```python
from build123d import *

# Parameters (mm, degrees)
EXTRUDE_THIN1_DEPTH = 4
SKETCH2_R           = 1.5
BOSS_EXTRUDE1_DEPTH = 4
FILLET1_DEPTH       = 4
FILLET1_2_DEPTH     = 4
SKETCH3_W           = 3.133113898
SKETCH3_H           = 7.459824135
CUT_EXTRUDE1_DEPTH  = 95.769370322


with BuildPart() as part:
    # Sketch1 → Extrude-Thin1 (new body)
    with BuildSketch(Plane.XY):
        Polygon((-70, -25.358547654), (30, 11.038475773), (-60, 63), (-70, 63), (-70, 61), (-60.535898385, 61), (25.285605056, 11.450931886), (-70.684040287, -23.479162412), align=None)
    extrude(amount=EXTRUDE_THIN1_DEPTH)

    # Sketch2 → Boss-Extrude1 (add)
    # profile 1 of 17: a face of its own
    with BuildSketch(Plane(origin=(0, 0, 0), x_dir=(-1, 0, 0), z_dir=(0, 0, -1))):
        with BuildLine():
            ThreePointArc((69.699771159, -19.718666382), (66.807539781, -16.271839247), (62.910846986, -18.521595881))
            ThreePointArc((62.910846986, -18.521595881), (62.703305352, -19.561418618), (62.816669308, -20.615673554))
            Line((62.816669308, -20.615673554), (68.214792437, -22.580429694))
            ThreePointArc((68.214792437, -22.580429694), (68.979296275, -21.845692505), (69.488695332, -20.915736884))
            ThreePointArc((69.488695332, -20.915736884), (69.646598295, -20.326435004), (69.699771159, -19.718666382))
        make_face()
        with Locations((66.199771159, -19.718666382)):
            Circle(SKETCH2_R, mode=Mode.SUBTRACT)
    # profile 2 of 17: a face of its own
    with BuildSketch(Plane(origin=(0, 0, 0), x_dir=(-1, 0, 0), z_dir=(0, 0, -1))):
        with BuildLine():
            ThreePointArc((69.488695332, -20.915736884), (68.979296275, -21.845692505), (68.214792437, -22.580429694))
            Line((68.214792437, -22.580429694), (68.804655045, -22.795122125))
            Line((68.804655045, -22.795122125), (69.488695332, -20.915736884))
        make_face()
    # profile 3 of 17: a face of its own
    with BuildSketch(Plane(origin=(0, 0, 0), x_dir=(-1, 0, 0), z_dir=(0, 0, -1))):
        with BuildLine():
            Line((62.910846986, -18.521595881), (62.2268067, -20.400981122))
            Line((62.2268067, -20.400981122), (62.816669308, -20.615673554))
            ThreePointArc((62.816669308, -20.615673554), (62.703305352, -19.561418618), (62.910846986, -18.521595881))
        make_face()
    # profile 4 of 17: a face of its own
    with BuildSketch(Plane(origin=(0, 0, 0), x_dir=(-1, 0, 0), z_dir=(0, 0, -1))):
        with BuildLine():
            ThreePointArc((22.71514012, -2.617659216), (19.822908742, 0.82916792), (15.926215947, -1.420588714))
            ThreePointArc((15.926215947, -1.420588714), (15.718674313, -2.460411452), (15.832038269, -3.514666388))
            Line((15.832038269, -3.514666388), (21.230161397, -5.479422527))
            ThreePointArc((21.230161397, -5.479422527), (21.994665236, -4.744685339), (22.504064292, -3.814729718))
            ThreePointArc((22.504064292, -3.814729718), (22.661967255, -3.225427838), (22.71514012, -2.617659216))
        make_face()
        with Locations((19.21514012, -2.617659216)):
            Circle(SKETCH2_R, mode=Mode.SUBTRACT)
    # profile 5 of 17: a face of its own
    with BuildSketch(Plane(origin=(0, 0, 0), x_dir=(-1, 0, 0), z_dir=(0, 0, -1))):
        with BuildLine():
            ThreePointArc((22.504064292, -3.814729718), (21.994665236, -4.744685339), (21.230161397, -5.479422527))
            Line((21.230161397, -5.479422527), (21.820024006, -5.694114959))
            Line((21.820024006, -5.694114959), (22.504064292, -3.814729718))
        make_face()
    # profile 6 of 17: a face of its own
    with BuildSketch(Plane(origin=(0, 0, 0), x_dir=(-1, 0, 0), z_dir=(0, 0, -1))):
        with BuildLine():
            Line((15.926215947, -1.420588714), (15.24217566, -3.299973956))
            Line((15.24217566, -3.299973956), (15.832038269, -3.514666388))
            ThreePointArc((15.832038269, -3.514666388), (15.718674313, -2.460411452), (15.926215947, -1.420588714))
        make_face()
    # profile 7 of 17: a face of its own
    with BuildSketch(Plane(origin=(0, 0, 0), x_dir=(-1, 0, 0), z_dir=(0, 0, -1))):
        with BuildLine():
            ThreePointArc((-18.249808849, 11.760273971), (-18.650603728, 13.386597315), (-19.761196061, 14.640450906))
            Line((-19.761196061, 14.640450906), (-22.499808851, 13.059312075))
            ThreePointArc((-22.499808851, 13.059312075), (-20.99980885, 13.059312077), (-20.249808849, 11.760273971))
            ThreePointArc((-20.249808849, 11.760273971), (-20.889444174, 10.531545919), (-22.262839017, 10.350735022))
            Line((-22.262839017, 10.350735022), (-19.291270082, 9.269172381))
            ThreePointArc((-19.291270082, 9.269172381), (-18.520653721, 10.410252801), (-18.249808849, 11.760273971))
        make_face()
    # profile 8 of 17: a face of its own
    with BuildSketch(Plane(origin=(0, 0, 0), x_dir=(-1, 0, 0), z_dir=(0, 0, -1))):
        with BuildLine():
            Line((-22.499808851, 13.059312075), (-25.238421636, 11.478173246))
            ThreePointArc((-25.238421636, 11.478173246), (-25.236490292, 11.455228871), (-25.234408046, 11.432297698))
            Line((-25.234408046, 11.432297698), (-22.262839017, 10.350735022))
            ThreePointArc((-22.262839017, 10.350735022), (-23.244100894, 11.62954033), (-22.499808851, 13.059312075))
        make_face()
    # profile 9 of 17: a face of its own
    with BuildSketch(Plane(origin=(0, 0, 0), x_dir=(-1, 0, 0), z_dir=(0, 0, -1))):
        with BuildLine():
            ThreePointArc((-18.249808849, 11.760273971), (-18.650603728, 13.386597315), (-19.761196061, 14.640450906))
            Line((-19.761196061, 14.640450906), (-22.499808851, 13.059312075))
            ThreePointArc((-22.499808851, 13.059312075), (-20.99980885, 13.059312077), (-20.249808849, 11.760273971))
            ThreePointArc((-20.249808849, 11.760273971), (-20.889444174, 10.531545919), (-22.262839017, 10.350735022))
            Line((-22.262839017, 10.350735022), (-19.291270082, 9.269172381))
            ThreePointArc((-19.291270082, 9.269172381), (-18.520653721, 10.410252801), (-18.249808849, 11.760273971))
        make_face()
    # profile 10 of 17: a face of its own
    with BuildSketch(Plane(origin=(0, 0, 0), x_dir=(-1, 0, 0), z_dir=(0, 0, -1))):
        with BuildLine():
            Line((-22.499808851, 13.059312075), (-25.238421636, 11.478173246))
            ThreePointArc((-25.238421636, 11.478173246), (-25.236490292, 11.455228871), (-25.234408046, 11.432297698))
            Line((-25.234408046, 11.432297698), (-22.262839017, 10.350735022))
            ThreePointArc((-22.262839017, 10.350735022), (-23.244100894, 11.62954033), (-22.499808851, 13.059312075))
        make_face()
    # profile 11 of 17: a face of its own
    with BuildSketch(Plane(origin=(0, 0, 0), x_dir=(-1, 0, 0), z_dir=(0, 0, -1))):
        with BuildLine():
            ThreePointArc((-25.234408046, 11.432297698), (-25.236490292, 11.455228871), (-25.238421636, 11.478173246))
            Line((-25.238421636, 11.478173246), (-25.285605056, 11.450931886))
            Line((-25.285605056, 11.450931886), (-25.234408046, 11.432297698))
        make_face()
    # profile 12 of 17: a face of its own
    with BuildSketch(Plane(origin=(0, 0, 0), x_dir=(-1, 0, 0), z_dir=(0, 0, -1))):
        with BuildLine():
            ThreePointArc((27.36379332, 37.517949192), (27.244533712, 38.42381585), (26.894882233, 39.267949192))
            ThreePointArc((26.894882233, 39.267949192), (26.231736995, 40.09532048), (25.351261913, 40.686140662))
            Line((25.351261913, 40.686140662), (20.376324727, 37.813859338))
            ThreePointArc((20.376324727, 37.813859338), (20.447752473, 36.75593546), (20.832704407, 35.767949192))
            ThreePointArc((20.832704407, 35.767949192), (24.769659978, 34.1372088), (27.36379332, 37.517949192))
        make_face()
        with Locations((23.86379332, 37.517949192)):
            Circle(SKETCH2_R, mode=Mode.SUBTRACT)
    # profile 13 of 17: a face of its own
    with BuildSketch(Plane(origin=(0, 0, 0), x_dir=(-1, 0, 0), z_dir=(0, 0, -1))):
        with BuildLine():
            Line((26.894882233, 39.267949192), (25.894882233, 41))
            Line((25.894882233, 41), (25.351261913, 40.686140662))
            ThreePointArc((25.351261913, 40.686140662), (26.231736995, 40.09532048), (26.894882233, 39.267949192))
        make_face()
    # profile 14 of 17: a face of its own
    with BuildSketch(Plane(origin=(0, 0, 0), x_dir=(-1, 0, 0), z_dir=(0, 0, -1))):
        with BuildLine():
            ThreePointArc((20.832704407, 35.767949192), (20.447752473, 36.75593546), (20.376324727, 37.813859338))
            Line((20.376324727, 37.813859338), (19.832704407, 37.5))
            Line((19.832704407, 37.5), (20.832704407, 35.767949192))
        make_face()
    # profile 15 of 17: a face of its own
    with BuildSketch(Plane(origin=(0, 0, 0), x_dir=(-1, 0, 0), z_dir=(0, 0, -1))):
        with BuildLine():
            ThreePointArc((61, 59), (64.5, 55.5), (68, 59))
            ThreePointArc((68, 59), (67.839385021, 60.048097173), (67.372281323, 61))
            Line((67.372281323, 61), (61.627718677, 61))
            ThreePointArc((61.627718677, 61), (61.160614979, 60.048097173), (61, 59))
        make_face()
        with Locations((64.5, 59)):
            Circle(SKETCH2_R, mode=Mode.SUBTRACT)
    # profile 16 of 17: a face of its own
    with BuildSketch(Plane(origin=(0, 0, 0), x_dir=(-1, 0, 0), z_dir=(0, 0, -1))):
        with BuildLine():
            Line((61, 61), (61, 59))
            ThreePointArc((61, 59), (61.160614979, 60.048097173), (61.627718677, 61))
            Line((61.627718677, 61), (61, 61))
        make_face()
    # profile 17 of 17: a face of its own
    with BuildSketch(Plane(origin=(0, 0, 0), x_dir=(-1, 0, 0), z_dir=(0, 0, -1))):
        with BuildLine():
            ThreePointArc((67.372281323, 61), (67.839385021, 60.048097173), (68, 59))
            Line((68, 59), (68, 61))
            Line((68, 61), (67.372281323, 61))
        make_face()
    extrude(amount=-BOSS_EXTRUDE1_DEPTH)

    # Fillet1: read off the stored shape, not the designer's step
    # Fillet1 outline → Fillet1 (cut)
    with BuildSketch(Plane.XY):
        with BuildLine():
            Line((30, 11.038475773), (24.428407585, 14.255236154))
            ThreePointArc((24.428407585, 14.255236154), (25.916991679, 11.395692714), (23.954468015, 8.83808208))
            Line((23.954468015, 8.83808208), (30, 11.038475773))
        make_face()
    extrude(amount=FILLET1_DEPTH, mode=Mode.SUBTRACT)

    # Fillet1 2 outline → Fillet1 2 (add)
    with BuildSketch(Plane.XY):
        with BuildLine():
            ThreePointArc((13.416857787, 18.303356317), (16.398283352, 15.667788657), (18.115840977, 12.078204963))
            ThreePointArc((18.115840977, 12.078204963), (15.801052244, 8.841405863), (12.407259711, 6.763597514))
            Line((12.407259711, 6.763597514), (19.291270082, 9.269172381))
            ThreePointArc((19.291270082, 9.269172381), (18.263127406, 12.06531907), (19.761196061, 14.640450906))
            Line((19.761196061, 14.640450906), (13.416857787, 18.303356317))
        make_face()
        with BuildLine():
            ThreePointArc((-69.488695332, -20.915736884), (-69.65911424, -20.25059255), (-69.696395151, -19.564976241))
            ThreePointArc((-69.696395151, -19.564976241), (-69.990650839, -21.572424943), (-70.684040287, -23.479162412))
            Line((-70.684040287, -23.479162412), (-68.804655045, -22.795122125))
            Line((-68.804655045, -22.795122125), (-69.488695332, -20.915736884))
        make_face()
        with BuildLine():
            Line((-62.2268067, -20.400981122), (-55.29724871, -17.878828277))
            ThreePointArc((-55.29724871, -17.878828277), (-59.906584574, -18.410948313), (-64.259910155, -16.80543119))
            ThreePointArc((-64.259910155, -16.80543119), (-63.448161827, -17.555648564), (-62.910846986, -18.521595881))
            Line((-62.910846986, -18.521595881), (-62.2268067, -20.400981122))
        make_face()
        with BuildLine():
            ThreePointArc((-22.504064292, -3.814729718), (-22.713356211, -2.729391821), (-22.573751348, -1.632910203))
            ThreePointArc((-22.573751348, -1.632910203), (-24.876585704, -5.661071418), (-28.749581995, -8.216267804))
            Line((-28.749581995, -8.216267804), (-21.820024006, -5.694114959))
            Line((-21.820024006, -5.694114959), (-22.504064292, -3.814729718))
        make_face()
        with BuildLine():
            Line((-15.24217566, -3.299973956), (-8.312617671, -0.777821111))
            ThreePointArc((-8.312617671, -0.777821111), (-12.921953535, -1.309941147), (-17.275279116, 0.295575976))
            ThreePointArc((-17.275279116, 0.295575976), (-16.463530787, -0.454641397), (-15.926215947, -1.420588714))
            Line((-15.926215947, -1.420588714), (-15.24217566, -3.299973956))
        make_face()
        with BuildLine():
            ThreePointArc((-70, 61), (-68.69628443, 59.445406029), (-67.733186639, 57.65966267))
            ThreePointArc((-67.733186639, 57.65966267), (-67.93264863, 58.316682078), (-68, 59))
            Line((-68, 59), (-68, 61))
            Line((-68, 61), (-70, 61))
        make_face()
        with BuildLine():
            ThreePointArc((-61.013092006, 58.697555558), (-60.842404557, 59.862852348), (-60.535898385, 61))
            Line((-60.535898385, 61), (-61, 61))
            Line((-61, 61), (-61, 59))
            ThreePointArc((-61, 59), (-61.003274533, 58.848636166), (-61.013092006, 58.697555558))
        make_face()
    extrude(amount=FILLET1_2_DEPTH)

    # Sketch3 → Cut-Extrude1 (cut, through all)
    with BuildSketch(Plane.XY.offset(4)):
        with Locations((-71.566556949, -21.628635587)):
            Rectangle(SKETCH3_W, SKETCH3_H)
    extrude(amount=-CUT_EXTRUDE1_DEPTH, mode=Mode.SUBTRACT)


solid = part.part
```
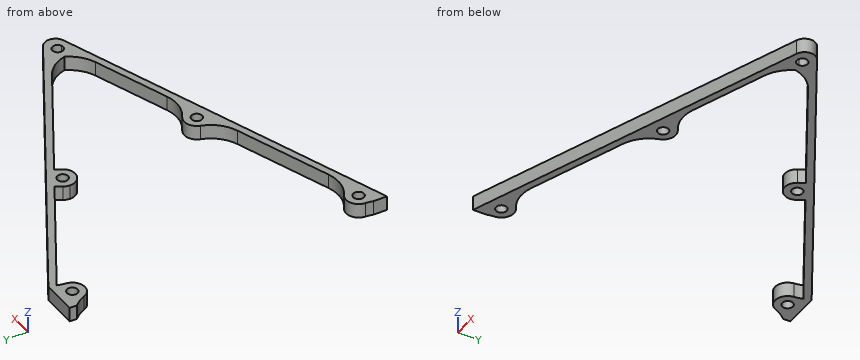
Geometry check sheet. Reference: the model listing, model coordinates, mm. Give positions to 0.01 mm unless a question says otherwise; leave off trailing zeros. Write each loop counter-clockwise with the first axis right and the second up, starting at its lowest first coordinate (ties: lowest second). Pieces come first, ordered by that corner, then holes. Notation, with made-up numbers: (38, -6) -> (49, -6) arc R26 cw to (49, 22) -> close; hole circle Ø10 at (-13, 45.25). An arc over 180 degrees is marked (long way). One line per question, with ' | ' between items.
Item 1: Sectioned sample at A-A, the plane x = -42.5. Record the boundary of the cut face in (y, z).
Determined:
outline: (-15.35, 0) -> (-13.22, 0) -> (-13.22, 4) -> (-15.35, 4) -> close; (50.59, 0) -> (52.9, 0) -> (52.9, 4) -> (50.59, 4) -> close
Item 2: Scan lines: line 1 along Y through (x, z) = (-19, 1.2); line 2 along Y through (x, z) = (-18, 1.9); line 3 along Y through (x, z) = (-33.5, 1.95). Record each from-to range of solid material in increasing order.
Determined:
line 1: -6.8 to -4.1, -1.13 to 0.88, 37.02 to 39.33 | line 2: -6.43 to -3.5, -1.74 to 0.66, 36.44 to 38.75 | line 3: -12.07 to -9.95, 45.39 to 47.7
Item 3: Sectioned sample at B-B, the plane z = 0.9. State how many separate pieces and enclosed holes the cut face has, plus the area to 3 significant figures.
Determined:
separate pieces: 1 | enclosed holes: 5 | area: 580 mm^2
Item 4: Sectioned sample at C-C, the plane x = 17. Record the boundary of the cut face in (y, z), plus the area to 3 significant figures.
Determined:
outline: (6.31, 0) -> (10.18, 0) -> (10.18, 4) -> (6.31, 4) -> close; (14.77, 0) -> (18.54, 0) -> (18.54, 4) -> (14.77, 4) -> close | area: 30.6 mm^2
Item 5: Depth check by flat-ended pin: pin 1 (2 mm diameter, centred on y = 21.5, z = 1.5, fed in from -X); pin 2 (2.5 mm diameter, centred on x = -64.5, y = 59, fed in from +Z); pin 3 (2 mm diameter, centred on x = -58.5, z = 1.5, fed in from -Y). Enter the tip coordinate at first touch or a pass-through.
Determined:
pin 1: x = 6.15 | pin 2: through | pin 3: y = -21.54
Item 6: Sectioned sample at D-D, the plane y = 42.5. Record the boundary of the cut face in (x, z).
Determined:
outline: (-28.49, 0) -> (-24.49, 0) -> (-24.49, 4) -> (-28.49, 4) -> close
